```python
from build123d import *
from OCP.BRepFilletAPI import BRepFilletAPI_MakeChamfer

# Parameters (mm, degrees)
BASE_EXTRUDE_DEPTH          = 3.302
BASE_EXTRUDE_DEPTH_BACK     = 3.302
SKETCH3_W                   = 7.62
SKETCH3_H                   = 9.398
CUT_EXTRUDE1_START          = -7.62
CUT_EXTRUDE1_DEPTH          = 7.62
SKETCH5_W                   = 3.5814
SKETCH5_H                   = 2.54
CUT_EXTRUDE2_DEPTH          = 0.127
BOSS_EXTRUDE1_START         = -9.906
SKETCH6_W                   = 0.635
SKETCH6_H                   = 0.635
BOSS_EXTRUDE1_DEPTH         = 13.716
CHAMFER1_SIZE               = 0.508
CHAMFER1_SIZE2              = 0.293293937
LPATTERN2_COUNT             = 3
LPATTERN2_PITCH             = 2.54
CHAMFER1_OF_LPATTERN2_SIZE  = 0.508
CHAMFER1_OF_LPATTERN2_SIZE2 = 0.293293937
LPATTERN3_COUNT             = 2
LPATTERN3_PITCH             = 2.54


# Read off the part's stored shape, not the designer's step: Cut-Extrude1
with BuildPart() as part:
    # Sketch3 → Base-Extrude (new, two sides: drawn at the far end of the back side and taken through both)
    with BuildSketch(Plane.XY.offset(-BASE_EXTRUDE_DEPTH_BACK)):
        with Locations((2.54, 4.699)):
            Rectangle(SKETCH3_W, SKETCH3_H)
    extrude(amount=BASE_EXTRUDE_DEPTH + BASE_EXTRUDE_DEPTH_BACK)

    # Cut-Extrude1 outline → Cut-Extrude1 (cut)
    with BuildSketch(Plane.ZY.offset(1.27).offset(CUT_EXTRUDE1_START)):
        with BuildLine():
            add(Edge.make_bspline(
                [(-2.286, 3.81), (-1.368133743, 5.298530644), (-0.381370103, 6.898794196), (-1.568138006, 6.86066242), (-1.651, 6.858)],
                knots=[0, 0, 0, 0, 0.930178433, 1, 1, 1, 1], degree=3))
            Line((-2.286, 3.81), (-2.286, 2.54))
            Line((-2.286, 2.54), (3.302, 2.54))
            Line((3.302, 2.54), (3.302, 9.398))
            Line((3.302, 9.398), (-1.651, 9.398))
            Line((-1.651, 9.398), (-1.651, 6.858))
        make_face()
    extrude(amount=CUT_EXTRUDE1_DEPTH, mode=Mode.SUBTRACT)

    # Sketch5 → Cut-Extrude2 (cut, symmetric)
    with BuildSketch(Plane(origin=(1.27, 0, 0), x_dir=(0, 0, -1), z_dir=(1, 0, 0))):
        with Locations((-1.5113, 1.27)):
            Rectangle(SKETCH5_W, SKETCH5_H)
        with BuildLine():
            Line((3.302, 2.54), (3.302, 9.398))
            Line((3.302, 9.398), (1.651, 9.398))
            Line((1.651, 9.398), (1.651, 6.858))
            add(Edge.make_bspline(
                [(2.286, 3.81), (1.368133743, 5.298530644), (0.381370103, 6.898794196), (1.568138006, 6.86066242), (1.651, 6.858)],
                knots=[0, 0, 0, 0, 0.930178433, 1, 1, 1, 1], degree=3))
            Line((2.286, 3.81), (2.286, 2.54))
            Line((2.286, 2.54), (3.302, 2.54))
        make_face()
    cut_extrude2 = extrude(amount=CUT_EXTRUDE2_DEPTH, both=True, mode=Mode.SUBTRACT)

    # Sketch6 → Boss-Extrude1 (add)
    with BuildSketch(Plane.XZ.offset(BOSS_EXTRUDE1_START)):
        Rectangle(SKETCH6_W, SKETCH6_H)
    boss_extrude1 = extrude(amount=BOSS_EXTRUDE1_DEPTH)

    # Chamfer1: one chamfer whose edges measure the first distance from different faces: ONE call of the kernel's chamfer builder (chamfer() names one face for all edges)
    chamfer1_edges_1 = [part.edges().sort_by_distance(p)[0] for p in [
        (-0.3175, 9.906, 0),
    ]]
    chamfer1_side_1 = [part.faces().sort_by_distance(p)[0] for p in [
        (-0.3175, 6.223, 0),
    ]]
    chamfer1_edges_2 = [part.edges().sort_by_distance(p)[0] for p in [
        (0, 9.906, -0.3175),
    ]]
    chamfer1_side_2 = [part.faces().sort_by_distance(p)[0] for p in [
        (0, 6.223, -0.3175),
    ]]
    chamfer1_edges_3 = [part.edges().sort_by_distance(p)[0] for p in [
        (0.3175, 9.906, 0),
    ]]
    chamfer1_side_3 = [part.faces().sort_by_distance(p)[0] for p in [
        (0.3175, 6.223, 0),
    ]]
    chamfer1_edges_4 = [part.edges().sort_by_distance(p)[0] for p in [
        (0, 9.906, 0.3175),
    ]]
    chamfer1_side_4 = [part.faces().sort_by_distance(p)[0] for p in [
        (0, 6.223, 0.3175),
    ]]
    chamfer1 = BRepFilletAPI_MakeChamfer(part.part.solid().wrapped)
    for e in chamfer1_edges_1:
        chamfer1.Add(CHAMFER1_SIZE, CHAMFER1_SIZE2, e.wrapped, chamfer1_side_1[0].wrapped)  # the first distance lies on this face
    for e in chamfer1_edges_2:
        chamfer1.Add(CHAMFER1_SIZE, CHAMFER1_SIZE2, e.wrapped, chamfer1_side_2[0].wrapped)  # the first distance lies on this face
    for e in chamfer1_edges_3:
        chamfer1.Add(CHAMFER1_SIZE, CHAMFER1_SIZE2, e.wrapped, chamfer1_side_3[0].wrapped)  # the first distance lies on this face
    for e in chamfer1_edges_4:
        chamfer1.Add(CHAMFER1_SIZE, CHAMFER1_SIZE2, e.wrapped, chamfer1_side_4[0].wrapped)  # the first distance lies on this face
    add(Compound.cast(chamfer1.Shape()), mode=Mode.REPLACE)

    # LPattern2: Boss-Extrude1 ×3
    with Locations(*[(i * LPATTERN2_PITCH, 0, 0) for i in range(1, LPATTERN2_COUNT)]):
        add(boss_extrude1)

    # Chamfer1 of LPattern2: one chamfer whose edges measure the first distance from different faces: ONE call of the kernel's chamfer builder (chamfer() names one face for all edges)
    chamfer1_of_lpattern2_edges_1 = [part.edges().sort_by_distance(p)[0] for p in [
        (2.2225, 9.906, 0),
    ]]
    chamfer1_of_lpattern2_side_1 = [part.faces().sort_by_distance(p)[0] for p in [
        (2.2225, 6.223, 0),
    ]]
    chamfer1_of_lpattern2_edges_2 = [part.edges().sort_by_distance(p)[0] for p in [
        (2.54, 9.906, -0.3175),
    ]]
    chamfer1_of_lpattern2_side_2 = [part.faces().sort_by_distance(p)[0] for p in [
        (2.54, 6.223, -0.3175),
    ]]
    chamfer1_of_lpattern2_edges_3 = [part.edges().sort_by_distance(p)[0] for p in [
        (2.8575, 9.906, 0),
    ]]
    chamfer1_of_lpattern2_side_3 = [part.faces().sort_by_distance(p)[0] for p in [
        (2.8575, 6.223, 0),
    ]]
    chamfer1_of_lpattern2_edges_4 = [part.edges().sort_by_distance(p)[0] for p in [
        (2.54, 9.906, 0.3175),
    ]]
    chamfer1_of_lpattern2_side_4 = [part.faces().sort_by_distance(p)[0] for p in [
        (2.54, 6.223, 0.3175),
    ]]
    chamfer1_of_lpattern2_edges_5 = [part.edges().sort_by_distance(p)[0] for p in [
        (4.7625, 9.906, 0),
    ]]
    chamfer1_of_lpattern2_side_5 = [part.faces().sort_by_distance(p)[0] for p in [
        (4.7625, 6.223, 0),
    ]]
    chamfer1_of_lpattern2_edges_6 = [part.edges().sort_by_distance(p)[0] for p in [
        (5.08, 9.906, -0.3175),
    ]]
    chamfer1_of_lpattern2_side_6 = [part.faces().sort_by_distance(p)[0] for p in [
        (5.08, 6.223, -0.3175),
    ]]
    chamfer1_of_lpattern2_edges_7 = [part.edges().sort_by_distance(p)[0] for p in [
        (5.3975, 9.906, 0),
    ]]
    chamfer1_of_lpattern2_side_7 = [part.faces().sort_by_distance(p)[0] for p in [
        (5.3975, 6.223, 0),
    ]]
    chamfer1_of_lpattern2_edges_8 = [part.edges().sort_by_distance(p)[0] for p in [
        (5.08, 9.906, 0.3175),
    ]]
    chamfer1_of_lpattern2_side_8 = [part.faces().sort_by_distance(p)[0] for p in [
        (5.08, 6.223, 0.3175),
    ]]
    chamfer1_of_lpattern2 = BRepFilletAPI_MakeChamfer(part.part.solid().wrapped)
    for e in chamfer1_of_lpattern2_edges_1:
        chamfer1_of_lpattern2.Add(CHAMFER1_OF_LPATTERN2_SIZE, CHAMFER1_OF_LPATTERN2_SIZE2, e.wrapped, chamfer1_of_lpattern2_side_1[0].wrapped)  # the first distance lies on this face
    for e in chamfer1_of_lpattern2_edges_2:
        chamfer1_of_lpattern2.Add(CHAMFER1_OF_LPATTERN2_SIZE, CHAMFER1_OF_LPATTERN2_SIZE2, e.wrapped, chamfer1_of_lpattern2_side_2[0].wrapped)  # the first distance lies on this face
    for e in chamfer1_of_lpattern2_edges_3:
        chamfer1_of_lpattern2.Add(CHAMFER1_OF_LPATTERN2_SIZE, CHAMFER1_OF_LPATTERN2_SIZE2, e.wrapped, chamfer1_of_lpattern2_side_3[0].wrapped)  # the first distance lies on this face
    for e in chamfer1_of_lpattern2_edges_4:
        chamfer1_of_lpattern2.Add(CHAMFER1_OF_LPATTERN2_SIZE, CHAMFER1_OF_LPATTERN2_SIZE2, e.wrapped, chamfer1_of_lpattern2_side_4[0].wrapped)  # the first distance lies on this face
    for e in chamfer1_of_lpattern2_edges_5:
        chamfer1_of_lpattern2.Add(CHAMFER1_OF_LPATTERN2_SIZE, CHAMFER1_OF_LPATTERN2_SIZE2, e.wrapped, chamfer1_of_lpattern2_side_5[0].wrapped)  # the first distance lies on this face
    for e in chamfer1_of_lpattern2_edges_6:
        chamfer1_of_lpattern2.Add(CHAMFER1_OF_LPATTERN2_SIZE, CHAMFER1_OF_LPATTERN2_SIZE2, e.wrapped, chamfer1_of_lpattern2_side_6[0].wrapped)  # the first distance lies on this face
    for e in chamfer1_of_lpattern2_edges_7:
        chamfer1_of_lpattern2.Add(CHAMFER1_OF_LPATTERN2_SIZE, CHAMFER1_OF_LPATTERN2_SIZE2, e.wrapped, chamfer1_of_lpattern2_side_7[0].wrapped)  # the first distance lies on this face
    for e in chamfer1_of_lpattern2_edges_8:
        chamfer1_of_lpattern2.Add(CHAMFER1_OF_LPATTERN2_SIZE, CHAMFER1_OF_LPATTERN2_SIZE2, e.wrapped, chamfer1_of_lpattern2_side_8[0].wrapped)  # the first distance lies on this face
    add(Compound.cast(chamfer1_of_lpattern2.Shape()), mode=Mode.REPLACE)

    # LPattern3: Cut-Extrude2 ×2
    with Locations(*[(i * LPATTERN3_PITCH, 0, 0) for i in range(1, LPATTERN3_COUNT)]):
        add(cut_extrude2, mode=Mode.SUBTRACT)


solid = part.part
```
Check sheet for the modelled part. Datum: model origin and axes. Units: mm. A direction names the side the tool comes from. Coordinates: 2 decimals unless noted, no trailing zeros. Order: outer loops, then holes, each group sorted by start corner. A loop starts at its lowest first (then second) coordinate and runs counter-clockwise, first axis right, second up. Notation, with made-up numbers: M 0.5,48.25 L 31.5,48.25 A31 ccw 31.5,86.25 Z; hole C 22.25,-4.75 d9. An arc over 180 degrees is marked long. One line per question, with ' | ' between items. Start each with the question number.
Item 1: Material ranges on line 1 (X direction, y = 6, z = -2.75); line 2 (X direction, y = 9, z = 0.25); line 3 (Y direction, x = 0.75, z = -0.5), recorded low to high.
Item 2: Sectioned sample at D-D on y = 1.75. Record the cut outline in (x, z), and give its area (3 significant figures).
Item 3: Sectioned sample at C-C on z = 0.75. Record the cut outline in (x, y).
Item 4: Gauge pin test, flat ends, axial feed: P1, Ø0.7, axis at x = 0.5, y = 8, coming from the +Z side; P2, Ø2, axis at x = 4.5, z = -2, coming from the +Y side; P3, Ø2, axis at x = 1.5, z = -1.5, coming from the -Y side. Record the tip position at first contact, or that the pin passes through.
Item 5: Sectioned sample at A-A on y = -1. Record the cut outline in (x, z), and give its area (3 significant figures).
Item 6: Mould release check, pull along Y, two halves, no side actions. Record for faces 1 (the flat face through (3, 9.398, -2)), 2 (the flat face through (3.937, 6, -2)), 3 (the flat face through (3, 3, -2.286)): pulls with the +Y half, pulls with the -Y half, needs draft (parallel to the pull), parting line crosses it, or undercut.
Item 7: Sectioned sample at B-B on y = 8. Record the cut outline in (x, z), and give its area (3 significant figures).
Item 8: Access from +Z, -Z, +X, -X, +Y, -Y to the whole of each face (thin tool, end or side, straight path). Record for faces 4 (the flat face through (5, 9.398, -2)), 5 (the flat face through (6.35, 2, -1)), 6 (the flat face through (0, 8, -1.651)), 7 (the flat face through (5, 3, -2.286)), 8 (the flat face through (3.937, 1, 2)).
Answer below:
1) line 1: x = -1.27 to 1.14, 1.4 to 3.68, 3.94 to 6.35 | line 2: x = -0.32 to 0.32, 2.22 to 2.86, 4.76 to 5.4 | line 3: y = 0 to 2.54
2) outline: M -1.27,-3.3 L 6.35,-3.3 L 6.35,3.3 L 3.94,3.3 L 3.94,-0.28 L 3.68,-0.28 L 3.68,3.3 L 1.4,3.3 L 1.4,-0.28 L 1.14,-0.28 L 1.14,3.3 L -1.27,3.3 Z | area: 48.5 mm^2
3) outline: M -1.27,0 L 1.14,0 L 1.14,2.54 L -1.27,2.54 Z; M 1.4,0 L 3.68,0 L 3.68,2.54 L 1.4,2.54 Z; M 3.94,0 L 6.35,0 L 6.35,2.54 L 3.94,2.54 Z
4) P1: stops at z = 0.32 | P2: stops at y = 9.4 | P3: stops at y = 0
5) outline: M -0.32,-0.32 L 0.32,-0.32 L 0.32,0.32 L -0.32,0.32 Z; M 2.22,-0.32 L 2.86,-0.32 L 2.86,0.32 L 2.22,0.32 Z; M 4.76,-0.32 L 5.4,-0.32 L 5.4,0.32 L 4.76,0.32 Z | area: 1.21 mm^2
6) face 1: pulls with the +Y half | face 2: needs draft | face 3: undercut
7) outline: M -1.27,-3.3 L 1.14,-3.3 L 1.14,-1.65 L -1.27,-1.65 Z; M -0.32,-0.32 L 0.32,-0.32 L 0.32,0.32 L -0.32,0.32 Z; M 1.4,-3.3 L 3.68,-3.3 L 3.68,-1.65 L 1.4,-1.65 Z; M 2.22,-0.32 L 2.86,-0.32 L 2.86,0.32 L 2.22,0.32 Z; M 3.94,-3.3 L 6.35,-3.3 L 6.35,-1.65 L 3.94,-1.65 Z; M 4.76,-0.32 L 5.4,-0.32 L 5.4,0.32 L 4.76,0.32 Z | area: 13.0 mm^2
8) face 4: -Z, +X, -X, +Y | face 5: +Z, -Z, +X, +Y, -Y | face 6: +X, -X, +Y | face 7: +X, -X | face 8: +Z, +Y, -Y
